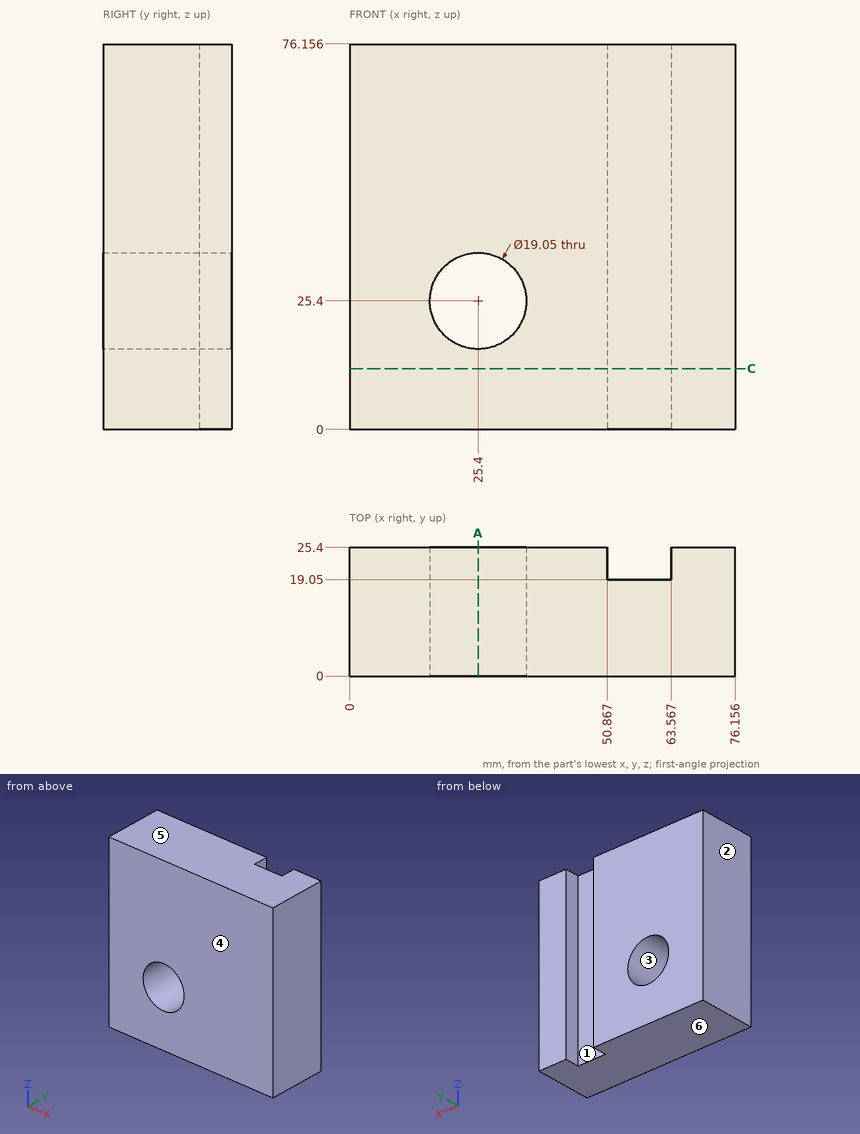
Job drawing, mm, ordinate dimensions from the low corner. One solid piece. A direction names the side the tool comes from. Round coordinates to 2 decimals unless told otherwise and drop trailing zeros. Order: outer loops, then holes, each group sorted by start corner. A loop starts at its lowest first (then second) coordinate and runs counter-clockwise, first axis right, second up. Notation, with made-up numbers: M -23.5,-31.5 L 32.5,-31.5 A24 cw 32.5,-18.5 Z; hole C 81.25,82 d6. An arc over 180 degrees is marked long. Write each question's results on one line, items separated by ' | '. Start each with the question number.
(1) Saw through at C-C, the plane z = 12. Give the cut face in (x, y), then the cut area to 3 significant figures.
(2) Which spindle directions (+Z, -Z, +X, -X, +Y, -Y) get a long thin tool onto all of the face, cutting with end or side? Do the marked faces 1 and 2. Say none if no direction does.
(3) Probe probe 1 along X at (y, z) = (18.25, 25.4) (1 decimal); probe 2 along Y at (x, z) = (55.5, 43); probe 3 along Z at (x, y) = (20, 16) (1 decimal). List the from-to ranges inside material, lowest first. Write a range as from..to.
(4) Saw through at A-A, the plane x = 25.4. Give the cut face in (y, z) (1 decimal).
(5) Drop flat-ended pins along their axis: pin 1 (2 mm diameter, centred on y = 3.5, z = 61.5, fed in from -X); pin 2 (4 mm diameter, centred on x = 55.5, z = 29, fed in from +Y); pin 3 (6 mm diameter, centred on x = 60, y = 22.5, fed in from -Z). Give the stop position or say it passes through.
(6) Two-plate mould, pull along Z, no slides. Class the marked faces 3, 4, 5 and 6: pulls with the +Z half, pulls with the -Z half, needs draft (parallel to the pull), parting line crosses it, or undercut.
Established:
1) outline: M 0,0 L 76.16,0 L 76.16,25.4 L 63.57,25.4 L 63.57,19.05 L 50.87,19.05 L 50.87,25.4 L 0,25.4 Z | area: 1,850 mm^2
2) face 1: +Z, -Z, +Y | face 2: +Z, -Z, -X, +Y, -Y
3) probe 1: x = 0..15.9, 34.9..76.2 | probe 2: y = 0..19.05 | probe 3: z = 0..17.6, 33.2..76.2
4) outline: M 0,0 L 25.4,0 L 25.4,15.9 L 0,15.9 Z; M 0,34.9 L 25.4,34.9 L 25.4,76.2 L 0,76.2 Z
5) pin 1: stops at x = 0 | pin 2: stops at y = 19.05 | pin 3: passes through
6) face 3: undercut | face 4: needs draft | face 5: pulls with the +Z half | face 6: pulls with the -Z half
